```python
from build123d import *

# Parameters (mm, degrees)
SKETCH1_R           = 2.9
BOSS_EXTRUDE1_DEPTH = 3.5
BOSS_EXTRUDE2_DEPTH = 23.076867
SKETCH3_R           = 2.25
CUT_EXTRUDE1_DEPTH  = 90.627435024


with BuildPart() as part:
    # Sketch1 → Boss-Extrude1 (new body)
    with BuildSketch(Plane.XY.offset(4.918735516)):
        with BuildLine():
            Line((23.684222564, -79.854061858), (27.751665024, -76.911614194))
            add(Edge.make_bspline(
                [(27.751665024, -76.911614194), (30.665612651, -71.996437575), (31.13217948, -67.256532156), (30.668059578, -56.517089881)],
                knots=[0.222415535, 0.222415535, 0.222415535, 0.222415535, 0.766682965, 0.766682965, 0.766682965, 0.766682965], degree=3))
            add(Edge.make_bspline(
                [(30.668059578, -56.517089881), (29.320428981, -45.88374403), (26.453494832, -35.554786486)],
                knots=[0, 0, 0, 1, 1, 1], degree=2))
            ThreePointArc((26.453494832, -35.554786486), (13.359197662, -30.130951008), (18.783033139, -43.225248178))
            add(Edge.make_bspline(
                [(18.783033139, -43.225248178), (19.322772584, -45.817228322), (25.294082339, -46.94058971), (23.583083134, -50.662102957)],
                knots=[0, 0, 0, 0, 1, 1, 1, 1], degree=3))
            Line((23.583083134, -50.662102957), (23.608661583, -58.04483203))
            Line((23.608661583, -58.04483203), (23.684222564, -79.854061858))
        make_face()
        with Locations((18.783033139, -35.554786486)):
            Circle(SKETCH1_R, mode=Mode.SUBTRACT)
    extrude(amount=-BOSS_EXTRUDE1_DEPTH)

    # Sketch2 → Boss-Extrude2 (add)
    with BuildSketch(Plane(origin=(0, 0, 1.418735516), x_dir=(-1, 0, 0), z_dir=(0, 0, -1))):
        with BuildLine():
            Line((-27.751665024, -76.911614194), (-23.684222564, -79.854061858))
            Line((-23.684222564, -79.854061858), (-23.608661583, -58.04483203))
            add(Edge.make_bspline(
                [(-23.608661583, -58.04483203), (-26.446360253, -54.336432943), (-30.668059578, -56.51708988)],
                knots=[0, 0, 0, 1, 1, 1], degree=2))
            add(Edge.make_bspline(
                [(-30.668059578, -56.51708988), (-31.132179479, -67.256532155), (-30.665612651, -71.996437575), (-27.751665024, -76.911614194)],
                knots=[0.222415535, 0.222415535, 0.222415535, 0.222415535, 0.766682965, 0.766682965, 0.766682965, 0.766682965], degree=3))
        make_face()
    extrude(amount=BOSS_EXTRUDE2_DEPTH)

    # Sketch3 → Cut-Extrude1 (cut, through all)
    with BuildSketch(Plane.XY.offset(4.918735516)):
        with Locations((27.143723241, -63.055671712)):
            Circle(SKETCH3_R)
    extrude(amount=-CUT_EXTRUDE1_DEPTH, mode=Mode.SUBTRACT)


solid = part.part
```
Source: CAD feature listing. Evaluate the final solid. Frame: model axes, mm. Round coordinates to 2 decimals unless told otherwise and drop trailing zeros. Loops run counter-clockwise (first coordinate to the right, second up) from the corner with the lowest first, then second, coordinate; pieces in that order, holes last.
1. Section query A-A on x = 13.5. Output: boundary loops of the cut face in (y, z).
2. Ray query, L1, parallel to Z at x = 14.5, y = -32.5; L2, parallel to X at y = -61.5, z = -6.75; L3, parallel to X at y = -62, z = -9.5. Return the intervals inside material, ascending.
3. Mould query, pull axis X, two halves, no side actions, for faces 1 (the flat face through (21, -39, 1.419)), 2 (the cylindrical face through (29.22, -63.92, -8.18)), 3 (the cylindrical face through (13.541, -29.955, 3.193)). Classes: released by +X, released by -X, zero draft, split by the parting line, or undercut.
4. Contact query for flat-ended pins moving along their axis: pin 1 (3 mm diameter, centred on y = -66.5, z = -11, fed in from -X); pin 2 (10 mm diameter, centred on x = 19.5, y = -43.5, fed in from -Z); pin 3 (5 mm diameter, centred on y = -72.5, z = -2, fed in from +X); pin 4 (6 mm diameter, centred on x = 27.14, y = -63.06, fed in from +Z). Output: stop coordinate, or through.
Answers below:
1. outline: (-41.12, 1.42) - (-29.99, 1.42) - (-29.99, 4.92) - (-41.12, 4.92) - close
2. L1: z = 1.42 to 4.92
2. L2: x = 23.62 to 25.52, 28.77 to 30.82
2. L3: x = 23.62 to 25.16, 29.13 to 30.82
3. face 1: zero draft
3. face 2: undercut
3. face 3: split by the parting line
4. pin 1: stops at x = 23.63
4. pin 2: stops at z = 1.42
4. pin 3: stops at x = 30.31
4. pin 4: stops at z = 4.92
